Design review of the part built by this model. Coordinates are the model's own, in mm. Face numbers are marked on the shaded views. A direction names the side the tool comes from. Coordinates: 2 decimals unless noted, no trailing zeros. Write each loop counter-clockwise with the first axis right and the second up, starting at its lowest first coordinate (ties: lowest second). Pieces come first, ordered by that corner, then holes. Notation, with made-up numbers: (77.5, -34.5) -> (116.5, -34.5) arc R18 ccw to (116.5, 0.5) -> close; hole circle Ø2 at (18, -13). An arc over 180 degrees is marked (long way). Answer in a Markdown table with one row per item. Add a question column.
Item 1: Clearance check with flat-ended pins moving along their axes: P1, Ø10, axis at x = 288, y = -536.5, coming from the +Z side; P2, Ø4, axis at x = 34, y = -211, coming from the +Z side. State where each tip first meets the part, or that it passes through.
Item 2: To check wall thickness, follow line 1 (Z direction, x = 205, y = -384); line 2 (X direction, y = -565, z = 99); line 3 (Z direction, x = 39, y = -50.5). State the ranges of each line that lie inside material, in increasing order.
Item 3: Draft analysis for pull direction Z (two halves, no side actions). For the marked faces 1, 2, 3 and 4, state which applies: released by +Z, released by -Z, zero draft, split by the parting line, or undercut.
Item 4: Take a section at C-C, the plane z = 221. Write out the cut boundary in (x, y).
Item 5: For the marked faces 5 and 6, list the 3-axis set-ups (+Z, -Z, +X, -X, +Y, -Y) from which the entire face can be reached by the end or side of a thin tool; tool diameter is ignored.
Item 6: Take a section at B-B, the plane y = -289. Write out the cut boundary in (x, z), and give its area (3 significant figures).
Item 7: Take a section at A-A, the plane x = 240. Write out the cut boundary in (y, z), and give its area (3 significant figures).
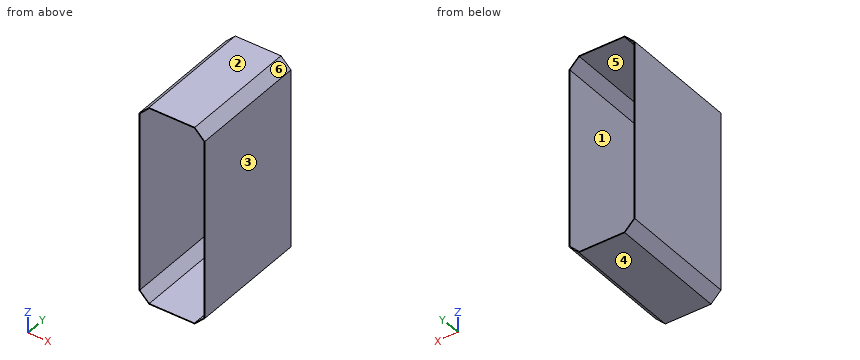
from build123d import *

# Parameters (mm, degrees)
F0_W     = 330
F0_H     = 1000
F1_DEPTH = 600
F2_SIZE  = 50
F3_T     = -4


with BuildPart() as f1:
    # F0 (on Front) → F1 (new body)
    with BuildSketch(Plane.XZ):
        with Locations((165, 500)):
            Rectangle(F0_W, F0_H)
    extrude(amount=F1_DEPTH)

    # F2
    f2_edges = [f1.edges().sort_by_distance(p)[0] for p in [
        (0, -300, 1000),
        (330, -300, 1000),
        (0, -300, 0),
        (330, -300, 0),
    ]]
    chamfer(f2_edges, length=F2_SIZE)

    # F3
    f3_openings = [f1.faces().sort_by_distance(p)[0] for p in [
        (165, -600, 500),
        (165, 0, 500),
    ]]
    offset(amount=F3_T, openings=f3_openings)


solid = f1.part
Answers:
| question | item | result |
|---|---|---|
| 1 | P1 | stops at z = 997 |
| 1 | P2 | stops at z = 986 |
| 2 | line 1 | z = 0 to 4, 996 to 1000 |
| 2 | line 2 | x = 0 to 4, 326 to 330 |
| 2 | line 3 | z = 11 to 16.66, 983.34 to 989 |
| 3 | face 1 | undercut |
| 3 | face 2 | released by +Z |
| 3 | face 3 | zero draft |
| 3 | face 4 | released by -Z |
| 4 | outline | (0, -600) -> (4, -600) -> (4, 0) -> (0, 0) -> close; (326, -600) -> (330, -600) -> (330, 0) -> (326, 0) -> close |
| 5 | face 5 | +Y, -Y |
| 5 | face 6 | +Z, +X, +Y, -Y |
| 6 | outline | (0, 50) -> (50, 0) -> (280, 0) -> (330, 50) -> (330, 950) -> (280, 1000) -> (50, 1000) -> (0, 950) -> close; hole (4, 51.66) -> (51.66, 4) -> (278.34, 4) -> (326, 51.66) -> (326, 948.34) -> (278.34, 996) -> (51.66, 996) -> (4, 948.34) -> close |
| 6 | area | 10,100 mm^2 |
| 7 | outline | (-600, 0) -> (0, 0) -> (0, 4) -> (-600, 4) -> close; (-600, 996) -> (0, 996) -> (0, 1000) -> (-600, 1000) -> close |
| 7 | area | 4,800 mm^2 |
